CAD build for the part. Positions are in the model's coordinates, mm. Face numbers are marked on the shaded views. A direction names the side the tool comes from. Coordinates: 2 decimals unless noted, no trailing zeros. Loops run counter-clockwise (first coordinate to the right, second up) from the corner with the lowest first, then second, coordinate; pieces in that order, holes last. Notation, with made-up numbers: (74, 86) -> (121, 86) arc R17 cw to (121, 98) -> close; hole circle Ø4 at (31, 88). An arc over 180 degrees is marked (long way). Write each question's results on one line, items separated by ' | '.
```python
from build123d import *

# Parameters (mm, degrees)
BOSS_EXTRUDE1_DEPTH                             = 3.18
SKETCH2_4_OUTSIDE_W                             = 40.864
SKETCH2_4_OUTSIDE_H                             = 68.924
SKETCH2_4_OUTSIDE_R                             = 5
CUT_EXTRUDE2_DEPTH                              = 3.18
FILLET6_R                                       = 3
CSK_FOR_M2_FLAT_HEAD_MACHINE_SCREW2_D           = 2.4
CSK_FOR_M2_FLAT_HEAD_MACHINE_SCREW2_CSINK_D     = 4.4
CSK_FOR_M2_FLAT_HEAD_MACHINE_SCREW2_CSINK_ANGLE = 90
M3X0_5_TAPPED_HOLE1_D                           = 3
M3X0_5_TAPPED_HOLE1_DEPTH                       = 3.328709071
M3X0_5_TAPPED_HOLE1_TIP                         = 0.901290929
SKETCH16_W                                      = 3.18
SKETCH16_H                                      = 12
BOSS_EXTRUDE2_DEPTH                             = 8.36
SKETCH18_W                                      = 6
SKETCH18_H                                      = 3.28
CUT_EXTRUDE3_DEPTH                              = 68.816439015


with BuildPart() as part:
    # Sketch2 → Boss-Extrude1 (new body)
    with BuildSketch(Plane(origin=(0, 0, 0), x_dir=(0, 0, -1), z_dir=(1, 0, 0))):
        Polygon((0, 54.73), (24, 54.73), (24, 15.53), (11.52, 15.53), (11.52, 14.38), (24.67, 14.38), (24.67, 10.38), (10.17, 10.38), (10.17, 0), (0, 0), (0, 17.7), (-2, 19.7), (-2, 29.7), (0, 31.7), align=None)
    extrude(amount=-BOSS_EXTRUDE1_DEPTH)

    # Sketch2<4> outside → Cut-Extrude2 (cut)
    # profile 1 of 3: a face of its own
    with BuildSketch(Plane(origin=(0, 0, 0), x_dir=(0, 0, -1), z_dir=(1, 0, 0))):
        with Locations((11.335, 27.365)):
            Rectangle(SKETCH2_4_OUTSIDE_W, SKETCH2_4_OUTSIDE_H)
        Polygon((0, 54.73), (24, 54.73), (24, 15.53), (11.52, 15.53), (11.52, 14.38), (24.67, 14.38), (24.67, 10.38), (10.17, 10.38), (10.17, 0), (0, 0), (0, 17.7), (-2, 19.7), (-2, 29.7), (0, 31.7), align=None, mode=Mode.SUBTRACT)
    # profile 2 of 3: a face of its own
    with BuildSketch(Plane(origin=(0, 0, 0), x_dir=(0, 0, -1), z_dir=(1, 0, 0))):
        with Locations((5, 24.7)):
            Circle(SKETCH2_4_OUTSIDE_R)
    # profile 3 of 3: a face of its own
    with BuildSketch(Plane(origin=(0, 0, 0), x_dir=(0, 0, -1), z_dir=(1, 0, 0))):
        with Locations((9, 40.810865899)):
            Circle(SKETCH2_4_OUTSIDE_R)
    extrude(amount=-CUT_EXTRUDE2_DEPTH, mode=Mode.SUBTRACT)

    # Fillet6
    fillet6_edges = [part.edges().sort_by_distance(p)[0] for p in [
        (-1.59, 31.7, 0),
        (-1.59, 29.7, 2),
        (-1.59, 19.7, 2),
        (-1.59, 17.7, 0),
        (-1.59, 0, 0),
    ]]
    fillet(fillet6_edges, radius=FILLET6_R)

    # CSK for M2 Flat Head Machine Screw2 (through all)
    with Locations(Plane.ZY.offset(3.18)):
        with Locations((-5.688374042, 46.403998609), (-15.499607993, 40.882251751), (-5.812017965, 35.146347336)):
            CounterSinkHole(CSK_FOR_M2_FLAT_HEAD_MACHINE_SCREW2_D / 2, CSK_FOR_M2_FLAT_HEAD_MACHINE_SCREW2_CSINK_D / 2, counter_sink_angle=CSK_FOR_M2_FLAT_HEAD_MACHINE_SCREW2_CSINK_ANGLE)

    # M3x0.5 Tapped Hole1
    with Locations(Plane(origin=(0, 0, 0), x_dir=(0, 0, -1), z_dir=(1, 0, 0))):
        with Locations((21.42, 12.38), (14.92, 12.38)):
            Hole(M3X0_5_TAPPED_HOLE1_D / 2, depth=M3X0_5_TAPPED_HOLE1_DEPTH)
            with Locations((0, 0, -(M3X0_5_TAPPED_HOLE1_DEPTH + M3X0_5_TAPPED_HOLE1_TIP / 2))):  # 118° drill point
                Cone(0, M3X0_5_TAPPED_HOLE1_D / 2, M3X0_5_TAPPED_HOLE1_TIP, mode=Mode.SUBTRACT)

    # Sketch16 → Boss-Extrude2 (add)
    with BuildSketch(Plane(origin=(0, 54.73, 0), x_dir=(1, 0, 0), z_dir=(0, 1, 0))):
        with Locations((-1.59, 12)):
            Rectangle(SKETCH16_W, SKETCH16_H)
    extrude(amount=BOSS_EXTRUDE2_DEPTH)

    # Sketch18 → Cut-Extrude3 (cut, through all)
    with BuildSketch(Plane(origin=(0, 0, 0), x_dir=(0, 0, -1), z_dir=(1, 0, 0))):
        with Locations((12, 59.55)):
            Rectangle(SKETCH18_W, SKETCH18_H)
    extrude(amount=-CUT_EXTRUDE3_DEPTH, mode=Mode.SUBTRACT)


solid = part.part
```
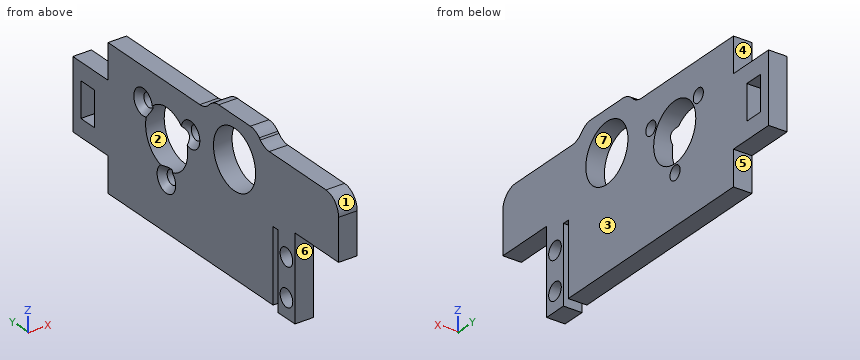
Q1. Cut at B-B on z = -12.25. Write the cut outline in (x, y), and give its area (3 significant figures).
Results are:
outline: (-3.18, 10.38) -> (0, 10.38) -> (0, 14.38) -> (-3.18, 14.38) -> close; (-3.18, 15.53) -> (0, 15.53) -> (0, 37.01) -> (-3.18, 37.01) -> close; (-3.18, 44.61) -> (0, 44.61) -> (0, 57.91) -> (-3.18, 57.91) -> close; (-3.18, 61.19) -> (0, 61.19) -> (0, 63.09) -> (-3.18, 63.09) -> close | area: 129 mm^2
Q2. Drop flat-ended pins along their axis: pin 1 (1.6 mm diameter, centred on x = -1.5, y = 28.5, fed in from -Z); pin 2 (1.6 mm diameter, centred on x = -1.5, z = -20, fed in from +Y); pin 3 (2.5 mm diameter, centred on y = 12.38, z = -14.92, fed in from +X); pin 4 (1.6 mm diameter, centred on x = -1, y = 58.5, fed in from +Z). Give the stop position or say it passes through.
Results are:
pin 1: z = -24 | pin 2: y = 54.73 | pin 3: through | pin 4: z = -6
Q3. Which spindle directions (+Z, -Z, +X, -X, +Y, -Y) get a long thin tool onto all of the face, cutting with end or side? Do the marked faces 4, 5, 6 and 7. Say none if no direction does.
Results are:
face 4: +Z, +X, -X, +Y | face 5: -Z, +X, -X, +Y | face 6: -Z, +X, -X, -Y | face 7: +X, -X
Q4. Cut at C-C on z = -21.25. Write the cut outline in (x, y), and give its area (3 significant figures).
Results are:
outline: (-3.18, 10.38) -> (0, 10.38) -> (0, 10.89) -> (-3.18, 10.89) -> close; (-3.18, 13.87) -> (0, 13.87) -> (0, 14.38) -> (-3.18, 14.38) -> close; (-3.18, 15.53) -> (0, 15.53) -> (0, 54.73) -> (-3.18, 54.73) -> close | area: 128 mm^2
Q5. Pull direction Z, two halves, no side cores. Call the marked faces 1, 2 and 3: +Z half, -Z half, draft (parallel to the pull), parting line (faces both ways), or undercut.
Results are:
face 1: +Z half | face 2: undercut | face 3: draft
Q6. Cut at D-D on x = -0.85. Give the number of separate pieces and of enclosed holes in the cut face, and give its area (3 significant figures).
Results are:
separate pieces: 1 | enclosed holes: 8 | area: 1,080 mm^2
Q7. Cut at A-A on y = 12.38. Write the cut outline in (x, z).
Results are:
outline: (-3.18, -24.67) -> (0, -24.67) -> (0, -22.92) -> (-3.18, -22.92) -> close; (-3.18, -19.92) -> (0, -19.92) -> (0, -16.42) -> (-3.18, -16.42) -> close; (-3.18, -13.42) -> (0, -13.42) -> (0, 0) -> (-3.18, 0) -> close
Q8. Wall check: L1, parallel to Y at x = -2.3, z = -14.92; L2, parallel to Y at x = -1.55, z = -21.5; L3, parallel to Y at x = -0.45, z = -16. Give the ranges that are in metal, low to high. Write a range as from..to.
Results are:
L1: 10.38..10.88, 13.88..14.38, 15.53..39.7, 42.07..57.91, 61.19..63.09 | L2: 10.38..10.88, 13.88..14.38, 15.53..54.73 | L3: 10.38..11.34, 13.42..14.38, 15.53..39.79, 41.97..63.09
